from build123d import *

# Parameters (mm, degrees)
SKETCH_1_R          = 25
EXTRUDE_1_DEPTH     = 20
SKETCH_2_R          = 17.5
CUT_EXTRUDE_1_DEPTH = 20
CUT_EXTRUDE_2_DEPTH = 38.5
SKETCH_4_R          = 21
CUT_EXTRUDE_3_DEPTH = 7


with BuildPart() as part:
    # 草图1 → 凸台-拉伸1 (new body)
    with BuildSketch(Plane(origin=(0, 0, 0), x_dir=(1, 0, 0), z_dir=(0, 1, 0))):
        Circle(SKETCH_1_R)
    extrude(amount=EXTRUDE_1_DEPTH)

    # 草图2 → 切除-拉伸1 (cut)
    with BuildSketch(Plane(origin=(0, 20, 0), x_dir=(1, 0, 0), z_dir=(0, 1, 0))):
        Circle(SKETCH_2_R)
    extrude(amount=-CUT_EXTRUDE_1_DEPTH, mode=Mode.SUBTRACT)

    # 草图3 → 切除-拉伸2 (cut, symmetric)
    with BuildSketch(Plane.XY):
        Polygon((-25, 8), (27.395295658, 17.238704287), (27.258418327, 39.934275436), (-34.828449814, 34.256390163), align=None)
    extrude(amount=CUT_EXTRUDE_2_DEPTH, both=True, mode=Mode.SUBTRACT)

    # 草图4 → 切除-拉伸3 (cut)
    with BuildSketch(Plane(origin=(-2.121922813, 12.034022275, 0), x_dir=(0.984807753, 0.173648178, 0), z_dir=(-0.173648178, 0.984807753, 0))):
        with Locations((2.154656893, 0)):
            Circle(SKETCH_4_R)
    extrude(amount=-CUT_EXTRUDE_3_DEPTH, mode=Mode.SUBTRACT)


solid = part.part
Here's how the part is built. I have some questions about the finished solid (model axes, mm). A direction names the side the tool comes from. Coordinates: 2 decimals unless noted, no trailing zeros. Order: outer loops, then holes, each group sorted by start corner. A loop starts at its lowest first (then second) coordinate and runs counter-clockwise, first axis right, second up. Notation, with made-up numbers: M -30,24 L 11,24 A26 cw 11,58 Z; hole C 54.5,-15 d7. An arc over 180 degrees is marked long. Answer as CSV lines item,"result". Start each with the question number.
1. On a 3-axis mill with a long thin cutter (end or side, diameter ignored), from which of +Z, -Z, +X, -X, +Y, -Y can I reach the whole of each face in a straight line? I mean faces 4 (the flat face through (17.97, 8.47, -0.1)), 5 (the cylindrical face through (16.166, 3.32, 6.703)). Say none if no direction works.
2. I need wall thicknesses on line 1 (Z direction, x = 0, y = 3.25); line 2 (X direction, y = 6.5, z = 0); line 3 (X direction, y = 5, z = -7). Which ranges of each line are inside material? Lowest first, please. Write a range as [from, to].
3. We'd pull the mould along Y, two halves only. Please class faces 1 (the cylindrical face through (20.325, 12.488, -6.308)), 2 (the flat face through (-17, 0, 5)), 3 (the flat face through (-20.487, 8.796, 3.82)): released by +Y, released by -Y, zero draft, split by the parting line, or undercut.
4. For pin 1 (1.5 mm diameter, centred on y = 11, z = -19.5, fed in from +X); pin 2 (3 mm diameter, centred on y = 3, z = -3, fed in from +X), each with a flat end and sliding along its axis, tell me the tip position at first contact or that it passes through.
5. I want a section at A-A, the plane z = 13.5. Write out the boundary of the cut face in (x, y), and give its area (3 significant figures).
6. I want a section at C-C, the plane z = 19. Write out the boundary of the cut face in (x, y).
7. I want a section at B-B, the plane z = 8.5. Write out the boundary of the cut face in (x, y).
Recorded:
1,face 4,"none"
1,face 5,"+Y, -Y"
2,line 1,"z = [-25, -17.5], [17.5, 25]"
2,line 2,"x = [-25, -20.28], [17.5, 25]"
2,line 3,"x = [-24, -18.8], [16.04, 24]"
3,face 1,"undercut"
3,face 2,"released by -Y"
3,face 3,"released by +Y"
4,pin 1,"stops at x = 16.54"
4,pin 2,"stops at x = 24.95"
5,outline,"M -21.04,0 L -11.14,0 L -11.14,3.34 L -14.63,2.72 L -15.84,9.61 L -21.04,8.7 Z; M 11.14,0 L 21.04,0 L 21.04,16.12 L 15.84,15.2 L 17.06,8.31 L 11.14,7.26 Z"
5,area,"179 mm2"
6,outline,"M -16.25,0 L 16.25,0 L 16.25,15.27 L 8.81,13.96 L 10.02,7.07 L -7.59,3.96 L -8.81,10.86 L -16.25,9.54 Z"
7,outline,"M -23.51,0 L -15.3,0 L -15.3,2.6 L -17.7,2.18 L -18.91,9.07 L -23.51,8.26 Z; M 15.3,0 L 23.51,0 L 23.51,16.55 L 18.91,15.74 L 20.13,8.85 L 15.3,8 Z"
